Here's the drawing with two shaded views (mm, measured from the low corner). I have some questions. A direction names the side the tool comes from. Coordinates: 2 decimals unless noted, no trailing zeros. Order: outer loops, then holes, each group sorted by start corner. A loop starts at its lowest first (then second) coordinate and runs counter-clockwise, first axis right, second up. Notation, with made-up numbers: (59, 6) -> (115, 6) arc R22 ccw to (115, 41) -> close; hole circle Ø8 at (-15.5, -40). An arc over 180 degrees is marked (long way). Answer in a Markdown table with one row per item. Add a question column.
1. Imagine slicing it at B-B on z = 0.5. Write out the boundary of the cut face in (x, y) (1 decimal), plus the area to 3 significant figures.
2. On a 3-axis mill with a long thin cutter (end or side, diameter ignored), from which of +Z, -Z, +X, -X, +Y, -Y can I reach the whole of each face in a straight line? I mean the marked faces 4 and 5. Say none if no direction works.
3. If I drill on line 1 along Y through (x, z) = (12.2, 6.3); line 2 along X through (y, z) = (9.5, 3); line 3 along Z through (x, y) = (6, 10.25), over which ranges is the centre line in solid material (lowest first)? Write a range as [from, to].
4. Will these pins go through, and if not, where does the flat tip stop? pin 1 (1 mm diameter, centred on x = 13.5, z = 1.5, fed in from +Y); pin 2 (3 mm diameter, centred on x = 7, z = 6.5, fed in from -Y) (1 decimal); pin 3 (7 mm diameter, centred on x = 12.2, y = 12.2, fed in from +Z); pin 4 (2 mm diameter, centred on x = 13.5, y = 3, fed in from -Z).
5. We'd pull the mould along X, two halves only. Please class the marked faces 1, 2 and 3: pulls with the +X half, pulls with the -X half, needs draft (parallel to the pull), parting line crosses it, or undercut.
6. Imagine slicing it at C-C on x = 15.25. Write out the boundary of the cut face in (y, z) (1 decimal).
7. Imagine slicing it at D-D on z = 6.25. Write out the boundary of the cut face in (x, y), plus the area to 3 significant figures.
8. Imagine slicing it at A-A on x = 12.2. Write out the boundary of the cut face in (y, z) (1 decimal).
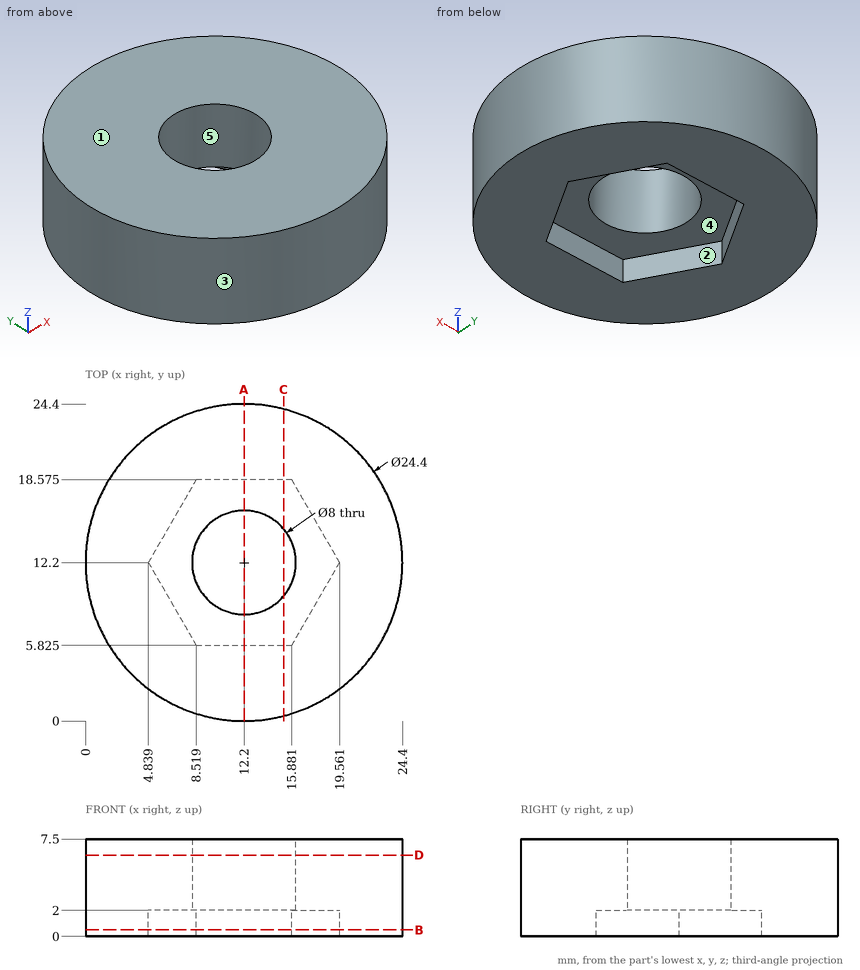
Answers follow:
| question | item | result |
|---|---|---|
| 1 | outline | circle Ø24.4 at (12.2, 12.2); hole (4.8, 12.2) -> (8.5, 5.8) -> (15.9, 5.8) -> (19.6, 12.2) -> (15.9, 18.6) -> (8.5, 18.6) -> close |
| 1 | area | 327 mm² |
| 2 | face 4 | -Z |
| 2 | face 5 | +Z, -Z |
| 3 | line 1 | y = [0, 8.2], [16.2, 24.4] |
| 3 | line 2 | x = [0.3, 9.25], [15.15, 24.1] |
| 3 | line 3 | z = [2, 7.5] |
| 4 | pin 1 | stops at y = 24.37 |
| 4 | pin 2 | stops at y = 0.6 |
| 4 | pin 3 | passes through |
| 4 | pin 4 | stops at z = 0 |
| 5 | face 1 | needs draft |
| 5 | face 2 | undercut |
| 5 | face 3 | parting line crosses it |
| 6 | outline | (0.4, 0) -> (5.8, 0) -> (5.8, 2) -> (9.6, 2) -> (9.6, 7.5) -> (0.4, 7.5) -> close; (14.8, 2) -> (18.6, 2) -> (18.6, 0) -> (24, 0) -> (24, 7.5) -> (14.8, 7.5) -> close |
| 7 | outline | circle Ø24.4 at (12.2, 12.2); hole circle Ø8 at (12.2, 12.2) |
| 7 | area | 417 mm² |
| 8 | outline | (0, 0) -> (5.8, 0) -> (5.8, 2) -> (8.2, 2) -> (8.2, 7.5) -> (0, 7.5) -> close; (16.2, 2) -> (18.6, 2) -> (18.6, 0) -> (24.4, 0) -> (24.4, 7.5) -> (16.2, 7.5) -> close |
